Design review of the part built by this model. Coordinates are the model's own, in mm. Face numbers are marked on the shaded views. Coordinates: 2 decimals unless noted, no trailing zeros. Write each loop counter-clockwise with the first axis right and the second up, starting at its lowest first coordinate (ties: lowest second). Pieces come first, ordered by that corner, then holes. Notation, with made-up numbers: (19.25, 42) -> (32.25, 42) arc R28 cw to (32.25, 61) -> close; hole circle Ø10 at (36.5, 56). An arc over 180 degrees is marked (long way). One line per question, with ' | ' between items. Start each with the question number.
Q1. Wall thickness on probe 1 along X at (y, z) = (200, 306); probe 2 along Z at (x, y) = (185.5, 147); probe 3 along Y at (x, z) = (218.5, 337): over which ranges is each line inside the solid? List them lowest first.
Q2. Add section A-A on z = 260. State the section outline as (x, y) points, and give its area (3 significant figures).
Q3. Add section B-B on y = 178. State the section outline as (x, z) points, and give its area (3 significant figures).
Q4. Draft analysis for pull direction X (two halves, no side actions). For the marked faces 1, 2, 3 and 4, state which applies: pulls with the +X half, pulls with the -X half, needs draft (parallel to the pull), parting line crosses it, or undercut.
Q5. Add section C-C on x = 184.5. State the section outline as (y, z) points, and give its area (3 significant figures).
Q6. Add section D-D on y = 110.5. State the section outline as (x, z) points, and give its area (3 significant figures).
Q7. For P1, Ø8, axis at x = 221.5, y = 161, coming from the -Z side; P2, Ø12, axis at x = 194.5, y = 121, coming from the +Z side; P3, Ø4, axis at x = 176, z = 324.5, coming from the -Y side; P4, Ø15.5, axis at y = 145.5, z = 343.5, coming from the -X side, all flat-tipped, find the tip position at first contact; note any pin that passes through.
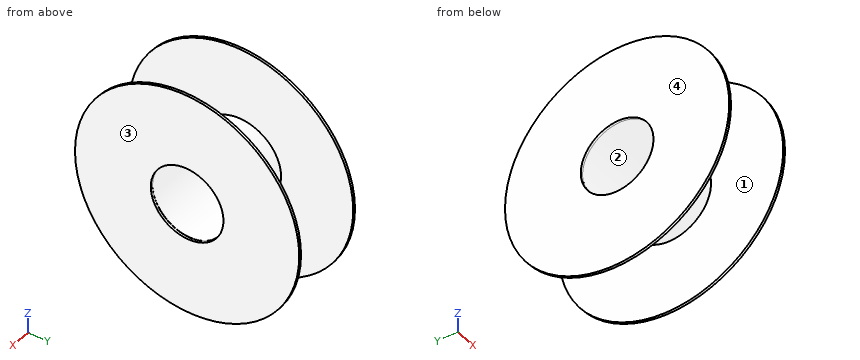
from build123d import *

# Parameters (mm, degrees)
SKETCH013_R   = 92.5
SKETCH013_R_2 = 30
PAD013_DEPTH  = 2
SKETCH014_R   = 33
SKETCH014_R_2 = 30
PAD014_DEPTH  = 58
SKETCH012_R   = 92.5
SKETCH012_R_2 = 30
PAD012_DEPTH  = 2


with BuildPart() as pad013:
    # Sketch013 → Pad013 (new body)
    with BuildSketch(Plane.YZ.offset(60)):
        with Locations((138.947021, 143.910721)):
            Circle(SKETCH013_R)
        with Locations((138.947021, 143.910721)):
            Circle(SKETCH013_R_2, mode=Mode.SUBTRACT)
    extrude(amount=PAD013_DEPTH)


with BuildPart() as pad014:
    # Sketch014 → Pad014 (new body)
    with BuildSketch(Plane.YZ.offset(2)):
        with Locations((138.95018, 144.130356)):
            Circle(SKETCH014_R)
        with Locations((138.95018, 144.130356)):
            Circle(SKETCH014_R_2, mode=Mode.SUBTRACT)
    extrude(amount=PAD014_DEPTH)


with BuildPart() as obj1:
    # Sketch012 → Pad012 (new body)
    with BuildSketch(Plane.YZ):
        with Locations((138.947021, 143.910721)):
            Circle(SKETCH012_R)
        with Locations((138.947021, 143.910721)):
            Circle(SKETCH012_R_2, mode=Mode.SUBTRACT)
    extrude(amount=PAD012_DEPTH)

    # Fusion014: union Pad013, Pad014
    add(pad013.part)
    add(pad014.part)


with BuildPart() as obj1_1:
    # Fusion014 placement: moved
    add(obj1.part.moved(Location((167, -8, 180))))


solid = obj1_1.part
Output values:
1) probe 1: x = 167 to 169, 227 to 229 | probe 2: z = 295.3 to 298.78, 349.48 to 352.96 | probe 3: y = 100.56 to 103.85, 158.05 to 161.34
2) outline: (167, 64.08) -> (169, 64.08) -> (169, 197.82) -> (167, 197.82) -> close; (227, 64.08) -> (229, 64.08) -> (229, 197.82) -> (227, 197.82) -> close | area: 535 mm2
3) outline: (167, 244.27) -> (169, 244.27) -> (169, 403.55) -> (167, 403.55) -> close; (227, 244.27) -> (229, 244.27) -> (229, 403.55) -> (227, 403.55) -> close | area: 637 mm2
4) face 1: undercut | face 2: undercut | face 3: pulls with the +X half | face 4: pulls with the -X half
5) outline: circle Ø66 at (130.95, 324.13); hole circle Ø60 at (130.95, 324.13) | area: 594 mm2
6) outline: (167, 233.7) -> (169, 233.7) -> (169, 298.23) -> (227, 298.23) -> (227, 233.7) -> (229, 233.7) -> (229, 301.96) -> (227, 301.96) -> (227, 302.18) -> (169, 302.18) -> (169, 301.96) -> (167, 301.96) -> close; (167, 345.86) -> (169, 345.86) -> (169, 346.08) -> (227, 346.08) -> (227, 345.86) -> (229, 345.86) -> (229, 414.12) -> (227, 414.12) -> (227, 350.03) -> (169, 350.03) -> (169, 414.12) -> (167, 414.12) -> close | area: 1,000 mm2
7) P1: stops at z = 303.87 | P2: stops at z = 356.89 | P3: stops at y = 97.95 | P4: stops at x = 167
